```python
from build123d import *

# Parameters (mm, degrees)
SKETCH1_W           = 25
SKETCH1_H           = 25
SKETCH1_W_2         = 23
SKETCH1_H_2         = 23
BOSS_EXTRUDE1_DEPTH = 200
SKETCH3_R           = 2
CUT_EXTRUDE1_DEPTH  = 25


with BuildPart() as part:
    # Sketch1 → Boss-Extrude1 (new body)
    with BuildSketch(Plane(origin=(0, 0, 0), x_dir=(1, 0, 0), z_dir=(0, 1, 0))):
        Rectangle(SKETCH1_W, SKETCH1_H)
        Rectangle(SKETCH1_W_2, SKETCH1_H_2, mode=Mode.SUBTRACT)
    extrude(amount=BOSS_EXTRUDE1_DEPTH)

    # Sketch3 → Cut-Extrude1 (cut)
    with BuildSketch(Plane(origin=(12.5, 0, 0), x_dir=(0, 0, -1), z_dir=(1, 0, 0))):
        with Locations((7.5, 190)):
            Circle(SKETCH3_R)
        with Locations((7.5, 180)):
            Circle(SKETCH3_R)
        with Locations((-7.5, 190)):
            Circle(SKETCH3_R)
        with Locations((-7.5, 180)):
            Circle(SKETCH3_R)
        with Locations((7.5, 170)):
            Circle(SKETCH3_R)
        with Locations((-7.5, 170)):
            Circle(SKETCH3_R)
    extrude(amount=-CUT_EXTRUDE1_DEPTH, mode=Mode.SUBTRACT)


solid = part.part
```
For this review, take the finished solid that the model builds, in its own axes (mm). A direction names the side the tool comes from. Round coordinates to 2 decimals unless told otherwise and drop trailing zeros. Order: outer loops, then holes, each group sorted by start corner. A loop starts at its lowest first (then second) coordinate and runs counter-clockwise, first axis right, second up. Notation, with made-up numbers: (85.5, 83) -> (136.5, 83) arc R19 ccw to (136.5, 94) -> close; hole circle Ø8 at (67, -3.5). An arc over 180 degrees is marked (long way). Use a Markdown table: item, result.
Item 1: For pin 1 (3.5 mm diameter, centred on y = 180, z = 7.5, fed in from -X), flat-tipped, find the tip position at first contact; note if it passes through.
Resolved:
| item | result |
|---|---|
| pin 1 | passes through |
Item 2: Take a section at C-C (y = 17). State the section outline as (x, z) points, plus the area to 3 significant figures.
Resolved:
| item | result |
|---|---|
| outline | (-12.5, -12.5) -> (12.5, -12.5) -> (12.5, 12.5) -> (-12.5, 12.5) -> close; hole (-11.5, -11.5) -> (11.5, -11.5) -> (11.5, 11.5) -> (-11.5, 11.5) -> close |
| area | 96.0 mm² |
Item 3: For line 1 along Y through (x, z) = (-11.8, 7.5); line 2 along Z through (x, y) = (-11.7, 170); line 3 along X through (y, z) = (10.5, 10), list the stretches that pass through material, from the lowest coordinate up. Write a range as [from, to].
Resolved:
| item | result |
|---|---|
| line 1 | y = [0, 168], [172, 178], [182, 188], [192, 200] |
| line 2 | z = [-12.5, -9.5], [-5.5, 5.5], [9.5, 12.5] |
| line 3 | x = [-12.5, -11.5], [11.5, 12.5] |
Item 4: Draft analysis for pull direction Y (two halves, no side actions). For faces 3 (the flat face through (-1, 0, 12)), 4 (the cylindrical face through (12.007, 188.226, 6.577)), 5 (the flat face through (11.5, 99, 0)), state which applies: +Y half, -Y half, draft (parallel to the pull), parting line (faces both ways), or undercut.
Resolved:
| item | result |
|---|---|
| face 3 | -Y half |
| face 4 | undercut |
| face 5 | draft |
Item 5: Take a section at A-A (z = 0). State the section outline as (x, y) points, plus the area to 3 significant figures.
Resolved:
| item | result |
|---|---|
| outline | (-12.5, 0) -> (-11.5, 0) -> (-11.5, 200) -> (-12.5, 200) -> close; (11.5, 0) -> (12.5, 0) -> (12.5, 200) -> (11.5, 200) -> close |
| area | 400 mm² |
Item 6: Take a section at D-D (z = 7.5). State how many separate pieces and enclosed holes the cut face has, plus the area to 3 significant figures.
Resolved:
| item | result |
|---|---|
| separate pieces | 8 |
| enclosed holes | 0 |
| area | 376 mm² |
Item 7: Take a section at B-B (x = 5.75). State the section outline as (y, z) points, plus the area to 3 significant figures.
Resolved:
| item | result |
|---|---|
| outline | (0, -12.5) -> (200, -12.5) -> (200, -11.5) -> (0, -11.5) -> close; (0, 11.5) -> (200, 11.5) -> (200, 12.5) -> (0, 12.5) -> close |
| area | 400 mm² |
Item 8: Machinability: for faces 1 (the flat face through (-11.5, 99, 0)), 2 (the flat face through (-1, 200, 12)), which of the approach directions +Z, -Z, +X, -X, +Y, -Y give a long, thin tool a straight path to every point of the face, cutting with its end or side? Answer none if there is none.
Resolved:
| item | result |
|---|---|
| face 1 | +Y, -Y |
| face 2 | +Z, -Z, +X, -X, +Y |
